Can you work these out from the model? Positions are in its coordinate system, mm. A direction names the side the tool comes from. Round coordinates to 2 decimals unless told otherwise and drop trailing zeros. Loops run counter-clockwise (first coordinate to the right, second up) from the corner with the lowest first, then second, coordinate; pieces in that order, holes last. Notation, with made-up numbers: M -3,-23.5 L 7,-23.5 A33 ccw 7,8.5 Z; hole C -3,74 d3. An arc over 180 degrees is marked long. Answer as CSV lines item,"result".
from build123d import *

# Parameters (mm, degrees)
SKETCH_1_W                  = 76
SKETCH_1_H                  = 20
SKETCH_1_W_2                = 18
SKETCH_1_W_3                = 10
SKETCH_1_H_2                = 18
SKETCH_1_W_4                = 20
SKETCH_1_H_3                = 52.041621827
EXTRUDE_1_DEPTH             = 5
HOLE_WIZARD_3_2_3_2_1_DEPTH = 5
SKETCH_8_W                  = 20
SKETCH_8_H                  = 110.041621827
EXTRUDE_2_DEPTH             = 2.2
HOLE_START                  = -2.2
HOLE_WIZARD_3_2_3_2_3_DEPTH = 7.2
RIB_1_REACH                 = 147.55
SKETCH_11_WALL_W            = 302.364540162
SKETCH_11_WALL_H            = 20
RIB_2_REACH                 = 113.533
SKETCH_12_WALL_W            = 234.330707354
SKETCH_12_WALL_H            = 20
RIB_3_REACH                 = 122.99
SKETCH_13_WALL_W            = 272.265137078
SKETCH_13_WALL_H            = 5
CHAMFER_1_SIZE              = 4


# Read off the part's stored shape, not the designer's step: Ø3.2 (3.2) 直径槽口1, Ø3.2 (3.2) 直径槽口3
with BuildPart() as part:
    # 草图1 → 凸台-拉伸1 (new body)
    with BuildSketch(Plane.XY):
        with Locations((-9.134530028, -25.635533007)):
            Rectangle(SKETCH_1_W, SKETCH_1_H)
        with Locations((-66.134530028, -25.635533007)):
            Rectangle(SKETCH_1_W_2, SKETCH_1_H)
        with Locations((-52.134530028, -25.635533007)):
            Rectangle(SKETCH_1_W_3, SKETCH_1_H)
        with Locations((-66.134530028, 12.364466993)):
            Rectangle(SKETCH_1_W_2, SKETCH_1_H)
        with Locations((-9.134530028, 12.364466993)):
            Rectangle(SKETCH_1_W, SKETCH_1_H)
        with Locations((-52.134530028, 12.364466993)):
            Rectangle(SKETCH_1_W_3, SKETCH_1_H)
        with Locations((-52.134530028, -6.635533007)):
            Rectangle(SKETCH_1_W_3, SKETCH_1_H_2)
        with Locations((-85.134530028, 12.364466993)):
            Rectangle(SKETCH_1_W_4, SKETCH_1_H)
        with Locations((-85.134530028, -6.635533007)):
            Rectangle(SKETCH_1_W_4, SKETCH_1_H_2)
        with Locations((-85.134530028, -25.635533007)):
            Rectangle(SKETCH_1_W_4, SKETCH_1_H)
        with Locations((-85.134530028, 48.385277907)):
            Rectangle(SKETCH_1_W_4, SKETCH_1_H_3)
    extrude(amount=EXTRUDE_1_DEPTH)

    # Ø3.2 (3.2) 直径槽口1 outline → Ø3.2 (3.2) 直径槽口1 (cut)
    with BuildSketch(Plane.XY):
        with BuildLine():
            Line((-36.134530028, 10.764466993), (23.865469972, 10.764466993))
            ThreePointArc((23.865469972, 10.764466993), (25.465469972, 12.364466993), (23.865469972, 13.964466993))
            Line((23.865469972, 13.964466993), (-36.134530028, 13.964466993))
            ThreePointArc((-36.134530028, 13.964466993), (-37.734530028, 12.364466993), (-36.134530028, 10.764466993))
        make_face()
        with BuildLine():
            Line((-36.134530028, -27.235533007), (23.865469972, -27.235533007))
            ThreePointArc((23.865469972, -27.235533007), (25.465469972, -25.635533007), (23.865469972, -24.035533007))
            Line((23.865469972, -24.035533007), (-36.134530028, -24.035533007))
            ThreePointArc((-36.134530028, -24.035533007), (-37.734530028, -25.635533007), (-36.134530028, -27.235533007))
        make_face()
    extrude(amount=HOLE_WIZARD_3_2_3_2_1_DEPTH, mode=Mode.SUBTRACT)

    # 草图8 → 凸台-拉伸2 (add)
    with BuildSketch(Plane(origin=(0, 0, 0), x_dir=(-1, 0, 0), z_dir=(0, 0, -1))):
        with Locations((85.134530028, 19.385277907)):
            Rectangle(SKETCH_8_W, SKETCH_8_H)
    extrude(amount=EXTRUDE_2_DEPTH)

    # Ø3.2 (3.2) 直径槽口3 outline → Ø3.2 (3.2) 直径槽口3 (cut)
    with BuildSketch(Plane.XY.offset(HOLE_START)):
        with BuildLine():
            Line((-83.534530028, -25.635533007), (-83.534530028, 54.364466993))
            ThreePointArc((-83.534530028, 54.364466993), (-85.134530028, 55.964466993), (-86.734530028, 54.364466993))
            Line((-86.734530028, 54.364466993), (-86.734530028, -25.635533007))
            ThreePointArc((-86.734530028, -25.635533007), (-85.134530028, -27.235533007), (-83.534530028, -25.635533007))
        make_face()
    extrude(amount=HOLE_WIZARD_3_2_3_2_3_DEPTH, mode=Mode.SUBTRACT)

    # 草图11 wall → 筋1 (add, up to next)
    with BuildSketch(Plane(origin=(-70.634530028, -35.635533007, -1.1), x_dir=(0.971399006497, 0, 0.237453090477), z_dir=(-0.237453090477, 0, 0.971399006497)), mode=Mode.PRIVATE) as rib_1_sk1:
        with Locations((0, 10)):
            Rectangle(SKETCH_11_WALL_W, SKETCH_11_WALL_H)
    rib_1_tool1 = extrude(rib_1_sk1.sketch, amount=RIB_1_REACH, mode=Mode.PRIVATE) - part.part
    add(rib_1_tool1.solids().sort_by_distance((-70.634530028, -35.635533007, -1.1))[0])

    # 草图12 wall → 筋2 (add, up to next)
    with BuildSketch(Plane(origin=(-70.634530028, 22.364466993, -1.1), x_dir=(0.971399006497, 0, 0.237453090477), z_dir=(0.237453090477, 0, -0.971399006497)), mode=Mode.PRIVATE) as rib_2_sk1:
        with Locations((0, 10)):
            Rectangle(SKETCH_12_WALL_W, SKETCH_12_WALL_H)
    rib_2_tool1 = extrude(rib_2_sk1.sketch, amount=-RIB_2_REACH, mode=Mode.PRIVATE) - part.part
    add(rib_2_tool1.solids().sort_by_distance((-70.634530028, 22.364466993, -1.1))[0])

    # 草图13 wall → 筋3 (add, up to next)
    with BuildSketch(Plane(origin=(-65.134530028, 32.364466993, 5), x_dir=(0.707106781187, -0.707106781187, 0), z_dir=(0.707106781187, 0.707106781187, 0)), mode=Mode.PRIVATE) as rib_3_sk1:
        with Locations((0, 2.5)):
            Rectangle(SKETCH_13_WALL_W, SKETCH_13_WALL_H)
    rib_3_tool1 = extrude(rib_3_sk1.sketch, amount=-RIB_3_REACH, mode=Mode.PRIVATE) - part.part
    add(rib_3_tool1.solids().sort_by_distance((-65.134530028, 32.364466993, 5))[0])

    # 倒角1
    chamfer_1_edges = [part.edges().sort_by_distance(p)[0] for p in [
        (-75.134530028, 74.40608882, 1.4),
        (-95.134530028, -35.635533007, 1.4),
        (-95.134530028, 74.40608882, 1.4),
    ]]
    chamfer(chamfer_1_edges, length=CHAMFER_1_SIZE)


solid = part.part
Item 1: If I drill on line 1 along Y through (x, z) = (4, 4); line 2 along X through (y, z) = (-10, 1.25); line 3 along X through (y, z) = (52.5, 2.5), over which ranges is the centre line in solid material (lowest first)? Write a range as from..to.
Output:
line 1,"y = -35.64..-27.24, -24.04..-15.64, 2.36..10.76, 13.96..22.36"
line 2,"x = -95.13..-86.73, -83.53..-75.13, -57.13..-47.13"
line 3,"x = -95.13..-86.73, -83.53..-75.13"
Item 2: If we section it at D-D on x = -40: Write out the boundary of the cut face in (y, z), then the cut area to 3 significant figures.
Output:
outline,"M -35.64,0 L -15.64,0 L -15.64,5 L -35.64,5 Z; M 2.36,0 L 22.36,0 L 22.36,5 L 2.36,5 Z"
area,"200 mm2"
Item 3: Will these pins go through, and if not, where does the flat tip stop? pin 1 (4 mm diameter, centred on x = -8, z = 3.5, fed in from +Y); pin 2 (0.7 mm diameter, centred on x = -69, z = -1.5, fed in from +Y); pin 3 (2 mm diameter, centred on y = 50.5, z = 3, fed in from +X); pin 4 (1.5 mm diameter, centred on y = -4.5, z = 2.5, fed in from +X).
Output:
pin 1,"stops at y = 22.36"
pin 2,"passes through"
pin 3,"stops at x = -75.13"
pin 4,"stops at x = -47.13"
Item 4: If we section it at B-B on y = -6.5: Write out the boundary of the cut face in (x, z).
Output:
outline,"M -95.13,-2.2 L -86.73,-2.2 L -86.73,5 L -95.13,5 Z; M -83.53,-2.2 L -75.13,-2.2 L -75.13,5 L -83.53,5 Z; M -57.13,0 L -47.13,0 L -47.13,5 L -57.13,5 Z"
Item 5: We'd pull the mould along X, two halves only. Please class faces 4 (the face through (-7, 10.764, 2)), 5 (the face through (-13, 22.364, 2)), 6 (the face through (-93.16, -33.61, 1.35)): released by +X, released by -X, zero draft, split by the parting line, or undercut.
Output:
face 4,"undercut"
face 5,"zero draft"
face 6,"released by -X"
Item 6: If we section it at C-C on y = 48: Write out the boundary of the cut face in (x, z).
Output:
outline,"M -95.13,-2.2 L -86.73,-2.2 L -86.73,5 L -95.13,5 Z; M -83.53,-2.2 L -75.13,-2.2 L -75.13,5 L -83.53,5 Z"
Item 7: On a 3-axis mill with a long thin cutter (end or side, diameter ignored), from which of +Z, -Z, +X, -X, +Y, -Y can I reach the whole of each face in a straight line? I mean faces 1 (the face through (-65.27, 32.5, 2.46)), 2 (the face through (25.465, -25.671, 2.465)), 3 (the face through (-10, 2.364, 2)). Say none if no direction works.
Output:
face 1,"+Z, -Z, +X, +Y"
face 2,"+Z, -Z"
face 3,"+Z, -Z, +X"
Item 8: If we section it at A-A on x = 9: Write out the boundary of the cut face in (y, z), then the cut area to 3 significant figures.
Output:
outline,"M -35.64,0 L -27.24,0 L -27.24,5 L -35.64,5 Z; M -24.04,0 L -15.64,0 L -15.64,5 L -24.04,5 Z; M 2.36,0 L 10.76,0 L 10.76,5 L 2.36,5 Z; M 13.96,0 L 22.36,0 L 22.36,5 L 13.96,5 Z"
area,"168 mm2"
